The drawing under review shows one solid part. Ordinate dimensions are in mm from its lowest x, y, z. Give positions to 0.01 mm unless a question says otherwise; leave off trailing zeros. Loops run counter-clockwise (first coordinate to the right, second up) from the corner with the lowest first, then second, coordinate; pieces in that order, holes last. Notation, with made-up numbers: M 20.5,15 L 70.5,15 A11 cw 70.5,30 Z; hole C 26.5,-34.75 d9. An arc over 180 degrees is marked long. Write item = value, one per line. Start each with the question number.
1. Wall thickness on line 1 along Y through (x, z) = (15, 63); line 2 along Y through (x, z) = (26.25, 98.5); line 3 along X through (y, z) = (22.5, 13): over which ranges is each line inside the solid? List them lowest first. Write a range as from..to.
2. We need section B-B on z = 63. Give the boundary of the cut face in (x, y), then the cut area to 3 significant figures.
3. We need section C-C on y = 15. Give the boundary of the cut face in (x, z).
4. For pin 1 (1.5 mm diameter, centred on y = 31.5, z = 71.5, fed in from -X); pin 2 (1.5 mm diameter, centred on y = 20, z = 31, fed in from +X); pin 3 (1.5 mm diameter, centred on y = 31, z = 54.5, fed in from +X), all flat-tipped, find the tip position at first contact; note any pin that passes through.
5. We need section A-A on x = 15. Give the boundary of the cut face in (y, z), then the cut area to 4 significant figures.
6. Draft analysis for pull direction X (two halves, no side actions). For the marked faces 1 and 2, state which applies: pulls with the +X half, pulls with the -X half, needs draft (parallel to the pull), parting line crosses it, or undercut.
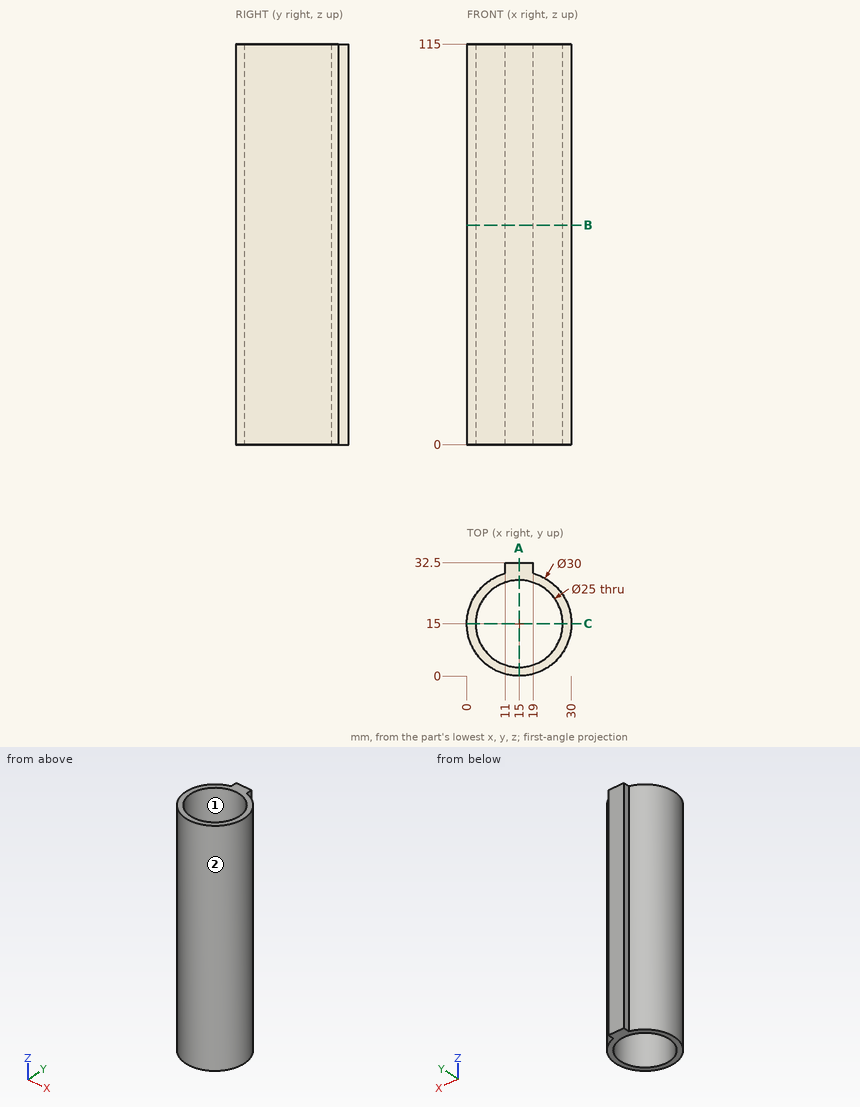
Final values:
q1.line_1 = 0..2.5, 27.5..32.5
q1.line_2 = 5.08..9.55, 20.45..24.92
q1.line_3 = 2.01..5, 25..27.99
q2.outline = M 11,29.46 A15 ccw long 19,29.46 L 19,32.5 L 11,32.5 Z; hole C 15,15 d25
q2.area = 237 mm²
q3.outline = M 0,0 L 2.5,0 L 2.5,115 L 0,115 Z; M 27.5,0 L 30,0 L 30,115 L 27.5,115 Z
q4.pin_1 = 11
q4.pin_2 = 29.39
q4.pin_3 = 19
q5.outline = M 0,0 L 2.5,0 L 2.5,115 L 0,115 Z; M 27.5,0 L 32.5,0 L 32.5,115 L 27.5,115 Z
q5.area = 862.5 mm²
q6.face_1 = undercut
q6.face_2 = parting line crosses it
